Job drawing, mm, ordinate dimensions from the low corner. One solid piece. A direction names the side the tool comes from. Round coordinates to 2 decimals unless told otherwise and drop trailing zeros. Loops run counter-clockwise (first coordinate to the right, second up) from the corner with the lowest first, then second, coordinate; pieces in that order, holes last.
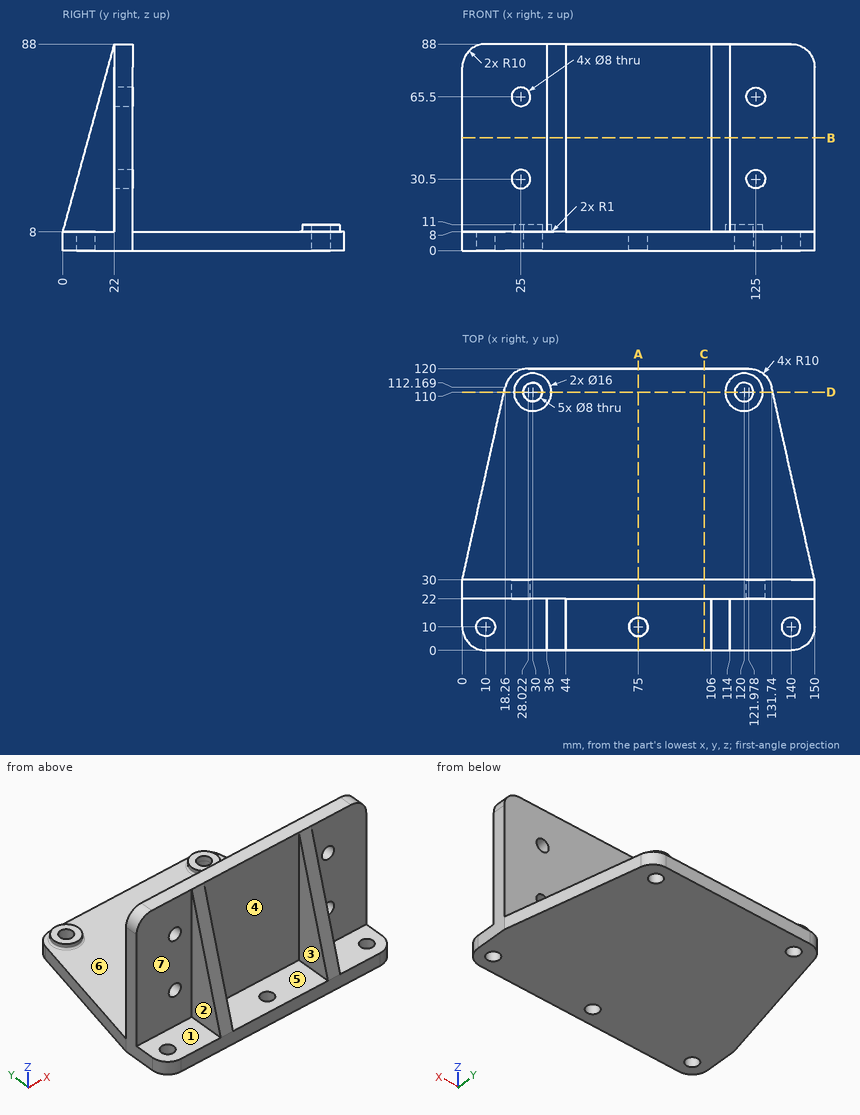
1) Wall check: line 1 along X through (y, z) = (24.5, 30.5); line 2 along Z through (x, y) = (25, 27); line 3 along Y through (x, z) = (75, 6). Give the ranges that are in metal, low to high.
Values:
line 1: x = 0 to 21, 29 to 121, 129 to 150
line 2: z = 0 to 26.5, 34.5 to 61.5, 69.5 to 88
line 3: y = 0 to 6, 14 to 120
2) Slice it at A-A, the plane x = 75. Give the cut face in (y, z), then the cut area to 3 significant figures.
Values:
outline: (0, 0) - (6, 0) - (6, 8) - (0, 8) - close; (14, 0) - (120, 0) - (120, 8) - (30, 8) - (30, 88) - (22, 88) - (22, 8) - (14, 8) - close
area: 1,540 mm2
3) Slice it at B-B, the plane z = 48. Give the cut face in (x, y), then the cut area to 3 significant figures.
Values:
outline: (0, 22) - (36, 22) - (36, 11) - (44, 11) - (44, 22) - (106, 22) - (106, 11) - (114, 11) - (114, 22) - (150, 22) - (150, 30) - (0, 30) - close
area: 1,380 mm2
4) Slice it at D-D, the plane y = 110. Give the cut face in (x, z).
Values:
outline: (17.78, 0) - (26, 0) - (26, 11) - (22, 11) - (22, 9) arc R1 cw to (21, 8) - (17.78, 8) - close; (34, 0) - (116, 0) - (116, 11) - (112, 11) - (112, 9) arc R1 cw to (111, 8) - (39, 8) arc R1 cw to (38, 9) - (38, 11) - (34, 11) - close; (124, 0) - (132.22, 0) - (132.22, 8) - (129, 8) arc R1 cw to (128, 9) - (128, 11) - (124, 11) - close
5) Mould opens along X. For the marked faces 1, 2, 3 and 4 say: released by +X, released by -X, zero draft, split by the parting line, or undercut.
Values:
face 1: zero draft
face 2: released by -X
face 3: undercut
face 4: undercut
6) Tool access for the marked faces 5, 6 and 7: list every direction of +Z, -Z, +X, -X, +Y, -Y with a clear straight run to the whole face (end or side of a thin tool).
Values:
face 5: +Z, -Y
face 6: +Z
face 7: +Z, -X, -Y
7) Slice it at C-C, the plane x = 103. Give the cut face in (y, z), then the cut area to 3 significant figures.
Values:
outline: (0, 0) - (120, 0) - (120, 8) - (30, 8) - (30, 88) - (22, 88) - (22, 8) - (0, 8) - close
area: 1,600 mm2
8) Drop flat-ended pins along their axis: pin 1 Ø4 at (x, y) = (45, 39) entering from +Z; pin 2 Ø12 at (x, z) = (92.5, 29) entering from -Y; pin 3 Ø13 at (x, y) = (120, 110) entering from +Z. Give the stop position or say it passes through.
Values:
pin 1: stops at z = 8
pin 2: stops at y = 22
pin 3: stops at z = 11
